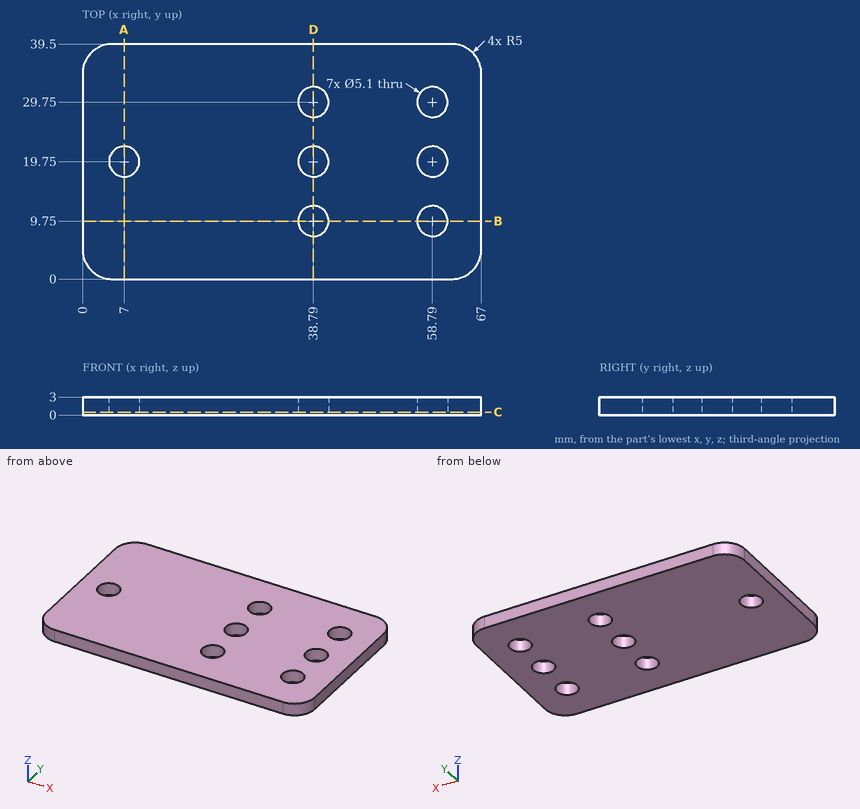
Could you check a few things on this drawing? It's one solid part, dimensions in mm from its lowest x, y, z. Give positions to 0.01 mm unless a question says otherwise; leave off trailing zeros. Order: outer loops, then holes, each group sorted by start corner. A loop starts at its lowest first (then second) coordinate and runs counter-clockwise, first axis right, second up. Notation, with made-up numbers: M 76.25,-26 L 99.25,-26 A12 cw 99.25,-7 Z; hole C -19,4 d5. An arc over 180 degrees is marked long. Use one line per item in the form item = value. Start each with the question number.
Item 1: If we section it at A-A (x = 7): Write out the boundary of the cut face in (y, z).
Item 2: If we section it at D-D (x = 38.79): Write out the boundary of the cut face in (y, z), then the cut area to 3 significant figures.
Item 3: If we section it at C-C (z = 0.5): Write out the boundary of the cut face in (x, y), then the cut area to 3 significant figures.
Item 4: Will these pins go through, and if not, where does the flat tip stop? pin 1 Ø4 at (x, y) = (58.79, 29.75) entering from +Z; pin 2 Ø1 at (y, z) = (7.5, 0.5) entering from -X.
Item 5: If we section it at B-B (y = 9.75): Write out the boundary of the cut face in (x, z), then the cut area to 3 significant figures.
Item 6: If I drill on line 1 along Y through (x, z) = (58.79, 2.1); line 2 along X through (y, z) = (30, 1.45); line 3 along Y through (x, z) = (7, 0.75), over which ranges is the centre line in solid material (lowest first)?
Outcome:
q1.outline = M 0,0 L 17.2,0 L 17.2,3 L 0,3 Z; M 22.3,0 L 39.5,0 L 39.5,3 L 22.3,3 Z
q2.outline = M 0,0 L 7.2,0 L 7.2,3 L 0,3 Z; M 12.3,0 L 17.2,0 L 17.2,3 L 12.3,3 Z; M 22.3,0 L 27.2,0 L 27.2,3 L 22.3,3 Z; M 32.3,0 L 39.5,0 L 39.5,3 L 32.3,3 Z
q2.area = 72.6 mm2
q3.outline = M 0,5 A5 ccw 5,0 L 62,0 A5 ccw 67,5 L 67,34.5 A5 ccw 62,39.5 L 5,39.5 A5 ccw 0,34.5 Z; hole C 7,19.75 d5.1; hole C 38.79,9.75 d5.1; hole C 38.79,19.75 d5.1; hole C 38.79,29.75 d5.1; hole C 58.79,9.75 d5.1; hole C 58.79,19.75 d5.1; hole C 58.79,29.75 d5.1
q3.area = 2,480 mm2
q4.pin_1 = through
q4.pin_2 = 0
q5.outline = M 0,0 L 36.24,0 L 36.24,3 L 0,3 Z; M 41.34,0 L 56.24,0 L 56.24,3 L 41.34,3 Z; M 61.34,0 L 67,0 L 67,3 L 61.34,3 Z
q5.area = 170 mm2
q6.line_1 = 0 to 7.2, 12.3 to 17.2, 22.3 to 27.2, 32.3 to 39.5
q6.line_2 = 0 to 36.25, 41.33 to 56.25, 61.33 to 67
q6.line_3 = 0 to 17.2, 22.3 to 39.5
